Check sheet for the modelled part. Datum: model origin and axes. Units: mm. Give positions to 0.01 mm unless a question says otherwise; leave off trailing zeros. Order: outer loops, then holes, each group sorted by start corner. A loop starts at its lowest first (then second) coordinate and runs counter-clockwise, first axis right, second up.
```python
from build123d import *

# Parameters (mm, degrees)
SKETCH1_W           = 40
SKETCH1_H           = 30
BOSS_EXTRUDE1_DEPTH = 14
FILLET1_R           = 5
CUT_EXTRUDE1_DEPTH  = 1


with BuildPart() as part:
    # Sketch1 → Boss-Extrude1 (new body)
    with BuildSketch(Plane(origin=(0, 0, 0), x_dir=(1, 0, 0), z_dir=(0, 1, 0))):
        Rectangle(SKETCH1_W, SKETCH1_H)
    extrude(amount=BOSS_EXTRUDE1_DEPTH)

    # Fillet1
    fillet1_edges = [part.edges().sort_by_distance(p)[0] for p in [
        (20, 7, 15),
        (-20, 7, 15),
        (-20, 7, -15),
        (20, 7, -15),
    ]]
    fillet(fillet1_edges, radius=FILLET1_R)

    # Sketch2 → Cut-Extrude1 (cut)
    with BuildSketch(Plane(origin=(0, 14, 0), x_dir=(1, 0, 0), z_dir=(0, 1, 0))):
        with BuildLine():
            Line((15, 12), (-15, 12))
            ThreePointArc((-15, 12), (-16.414213562, 11.414213562), (-17, 10))
            Line((-17, 10), (-17, -10))
            ThreePointArc((-17, -10), (-16.414213562, -11.414213562), (-15, -12))
            Line((-15, -12), (15, -12))
            ThreePointArc((15, -12), (16.414213562, -11.414213562), (17, -10))
            Line((17, -10), (17, 10))
            ThreePointArc((17, 10), (16.414213562, 11.414213562), (15, 12))
        make_face()
        with BuildLine():
            Line((15, 11), (-15, 11))
            ThreePointArc((-15, 11), (-15.707106781, 10.707106781), (-16, 10))
            Line((-16, 10), (-16, -10))
            ThreePointArc((-16, -10), (-15.707106781, -10.707106781), (-15, -11))
            Line((-15, -11), (15, -11))
            ThreePointArc((15, -11), (15.707106781, -10.707106781), (16, -10))
            Line((16, -10), (16, 10))
            ThreePointArc((16, 10), (15.707106781, 10.707106781), (15, 11))
        make_face(mode=Mode.SUBTRACT)
    extrude(amount=-CUT_EXTRUDE1_DEPTH, mode=Mode.SUBTRACT)


solid = part.part
```
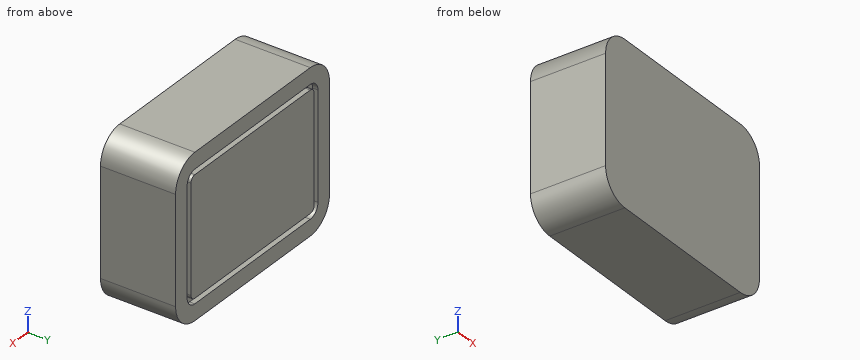
Q1. Material ranges on line 1 (Y direction, x = -4, z = 11.25); line 2 (X direction, y = 12.5, z = 12.75); line 3 (Z direction, x = 16, y = 3.5), recorded low to high.
Q2. Sectioned sample at B-B, the plane x = 16.5. Record the cut outline in (y, z), plus the area to 3 significant figures.
Q3. Sectioned sample at A-A, the plane y = 8. Record the cut outline in (x, z), plus the area to 3 significant figures.
Filled in:
1. line 1: y = 0 to 13
1. line 2: x = -19.18 to 19.18
1. line 3: z = -14.9 to 14.9
2. outline: (0, -14.77) - (14, -14.77) - (14, -11.32) - (13, -11.32) - (13, 11.32) - (14, 11.32) - (14, 14.77) - (0, 14.77) - close
2. area: 391 mm2
3. outline: (-20, -10) arc R5 ccw to (-15, -15) - (15, -15) arc R5 ccw to (20, -10) - (20, 10) arc R5 ccw to (15, 15) - (-15, 15) arc R5 ccw to (-20, 10) - close
3. area: 1,180 mm2
